from build123d import *

# Parameters (mm, degrees)
F0_R     = 1.0540994518
F1_DEPTH = 25.3238
F2_W     = 9.8913477779
F2_H     = 12.7
F3_DEPTH = 38.1
F4_W     = 37.0259946046
F4_H     = 12.7
F5_DEPTH = 25.4


with BuildPart() as f1:
    # F0 (on Front) → F1 (new body)
    with BuildSketch(Plane.XZ):
        with BuildLine():
            Line((-29.976574955, 27.7315109247), (-1.7824433728, -0.4626206574))
            ThreePointArc((-1.7824433728, -0.4626206574), (1.3021371376, -1.3021371376), (0.4626206574, 1.7824433728))
            Line((0.4626206574, 1.7824433728), (-57.9090441295, 60.1541081598))
            ThreePointArc((-57.9090441295, 60.1541081598), (-60.9187704252, 61.0135591282), (-60.2099135505, 57.9648495203))
            Line((-60.2099135505, 57.9648495203), (-32.5449282056, 30.2998641753))
            ThreePointArc((-32.5449282056, 30.2998641753), (-34.4523430384, 25.8240960919), (-29.976574955, 27.7315109247))
        make_face()
        with Locations((-32.5981950693, 27.678244061)):
            Circle(F0_R, mode=Mode.SUBTRACT)
        with Locations((0.0063811123, 0.0245859565)):
            Circle(F0_R, mode=Mode.SUBTRACT)
        with Locations((-59.6669015458, 59.6978686146)):
            Circle(F0_R, mode=Mode.SUBTRACT)
    extrude(amount=F1_DEPTH)

    # F2 (on Top) → F3 (cut)
    with BuildSketch(Plane.XY):
        with Locations((-32.6549597085, -12.7)):
            Rectangle(F2_W, F2_H)
    extrude(amount=F3_DEPTH, mode=Mode.SUBTRACT)

    # F4 (on face) → F5 (cut)
    with BuildSketch(Plane(origin=(1.1225320151, 0, 1.1225320151), x_dir=(0.7071067812, 0, -0.7071067812), z_dir=(0.7071067812, 0, 0.7071067812))):
        with Locations((-22.2613505073, -12.7)):
            Rectangle(F4_W, F4_H)
    extrude(amount=-F5_DEPTH, mode=Mode.SUBTRACT)


solid = f1.part
Here's how the part is built. I have some questions about the finished solid (model axes, mm). A direction names the side the tool comes from. Give positions to 0.01 mm unless a question says otherwise; leave off trailing zeros. Order: outer loops, then holes, each group sorted by start corner. A loop starts at its lowest first (then second) coordinate and runs counter-clockwise, first axis right, second up. Notation, with made-up numbers: M 44,-17 L 50,-17 A31 cw 50,15 Z; hole C 12,38.5 d11. An arc over 180 degrees is marked long. Answer as a JSON object with one key per item and string values. Group by question number.
1) Suppose I cut it at B-B, the plane x = -11.5. Write out the boundary of the cut face in (y, z).
2) Suppose I cut it at C-C, the plane x = -44.5. Write out the boundary of the cut face in (y, z), plus the area to 3 significant figures.
3) On a 3-axis mill with a long thin cutter (end or side, diameter ignored), from which of +Z, -Z, +X, -X, +Y, -Y can I reach the whole of each face in a straight line? I mean faces 1 (the cylindrical face through (-31.624, -3.131, 27.275)), 2 (the flat face through (-37.601, -13, 37)). Say none if no direction works.
4) I'm going to push flat-ended pins straight in: pin 1 Ø12 at (x, y) = (-34, -21) entering from +Z; pin 2 Ø2 at (x, y) = (-32.5, -3.5) entering from -Z; pin 3 Ø3 at (y, z) = (-9, 38.5) entering from -X. Where does each tip first touch, or does it pass through?
5) We'd pull the mould along Y, two halves only. Please class faces 3 (the flat face through (-32, 0, 32)), 4 (the cylindrical face through (-0.13, -12.48, 1.07)), 5 (the flat face through (-2.6, -12.8, 2.7)), 6 (the flat face through (-37, -13, 38.1)): pulls with the +Y half, pulls with the -Y half, needs draft (parallel to the pull), parting line crosses it, or undercut.
6) Suppose I cut it at A-A, the plane z = 23.5. Write out the boundary of the cut face in (x, y), plus the area to 3 significant figures.
7) Suppose I cut it at D-D, the plane z = 55. Write out the boundary of the cut face in (x, y), plus the area to 3 significant figures.
8) Please list where these lines run through material, in increasing order: L1, parallel to Y at x = -32.5, z = 30; L2, parallel to X at y = -22, z = 31; L3, parallel to Z at x = -51, y = -5.5. Write a range as [from, to].
Results found:
{
 "1": {"outline": "M -25.32,9.25 L -19.05,9.25 L -19.05,13.75 L -25.32,13.75 Z; M -6.35,9.25 L 0,9.25 L 0,13.75 L -6.35,13.75 Z"},
 "2": {"outline": "M -25.32,42.25 L 0,42.25 L 0,46.75 L -25.32,46.75 Z", "area": "114 mm²"},
 "3": {"face 1": "+Y, -Y", "face 2": "-Z, +X"},
 "4": {"pin 1": "z = 42.25", "pin 2": "z = 25.06", "pin 3": "x = -42.25"},
 "5": {"face 3": "pulls with the +Y half", "face 4": "needs draft", "face 5": "undercut", "face 6": "undercut"},
 "6": {"outline": "M -25.75,-25.32 L -21.25,-25.32 L -21.25,-19.05 L -25.75,-19.05 Z; M -25.75,-6.35 L -21.25,-6.35 L -21.25,0 L -25.75,0 Z", "area": "56.7 mm²"},
 "7": {"outline": "M -57.25,-25.32 L -52.75,-25.32 L -52.75,0 L -57.25,0 Z", "area": "114 mm²"},
 "8": {"L1": "[-25.32, -19.05], [-6.35, 0]", "L2": "[-33.25, -28.75]", "L3": "[48.75, 53.25]"}
}
